Input: part model. Units: mm. Frame: model coordinates. A direction names the side the tool comes from. Give positions to 0.01 mm unless a question says otherwise; leave off trailing zeros. Write each loop counter-clockwise with the first axis right and the second up, starting at its lowest first coordinate (ties: lowest second). Pieces come first, ordered by that corner, then holes. Notation, with made-up numbers: (85, 30.5) - (106, 30.5) arc R15 ccw to (106, 50.5) - close; hole circle Ø8 at (70.5, -25). An arc over 180 degrees is marked (long way). Answer as CSV lines item,"result".
```python
from build123d import *

# Parameters (mm, degrees)
SKETCH1_R           = 6
BOSS_EXTRUDE1_DEPTH = 10
SKETCH2_W           = 6.574952472
SKETCH2_H           = 6.574952471
BOSS_EXTRUDE2_DEPTH = 60
CUT_EXTRUDE1_DEPTH  = 72.85269654


with BuildPart() as part:
    # Sketch1 → Boss-Extrude1 (new body)
    with BuildSketch(Plane(origin=(0, 0, 0), x_dir=(1, 0, 0), z_dir=(0, 1, 0))):
        with Locations(Location((0, 0, 0), (0, 0, 270))):
            Circle(SKETCH1_R)
        with BuildLine():
            Line((-3.287476236, 2.45), (3.287476236, 2.45))
            ThreePointArc((3.287476236, 2.45), (0, -4.1), (-3.287476236, 2.45))
        make_face(mode=Mode.SUBTRACT)
    boss_extrude1 = extrude(amount=BOSS_EXTRUDE1_DEPTH)

    # Sketch2 → Boss-Extrude2 (add)
    with BuildSketch(Plane.XY.offset(-2.45)):
        with Locations((0, 3.287476236)):
            Rectangle(SKETCH2_W, SKETCH2_H)
    extrude(amount=-BOSS_EXTRUDE2_DEPTH)

    # Mirror1: Boss-Extrude1 across plane
    add(boss_extrude1.mirror(Plane(origin=(0, 0, -32.45), x_dir=(1, 0, 0), z_dir=(0, 0, -1))))

    # Sketch3 → Cut-Extrude1 (cut, through all)
    with BuildSketch(Plane(origin=(0, 10, 0), x_dir=(1, 0, 0), z_dir=(0, 1, 0))):
        with BuildLine():
            Line((-3.297499052, 62.43), (3.297499052, 62.43))
            ThreePointArc((3.297499052, 62.43), (0, 69.02), (-3.297499052, 62.43))
        make_face()
    extrude(amount=-CUT_EXTRUDE1_DEPTH, mode=Mode.SUBTRACT)


solid = part.part
```
Item 1: Contact query for flat-ended pins moving along their axis: pin 1 (1 mm diameter, centred on y = 6, z = -17, fed in from -X); pin 2 (5 mm diameter, centred on x = 1, z = -23.5, fed in from +Y); pin 3 (5.5 mm diameter, centred on y = 2, z = -43.5, fed in from +X). Output: stop coordinate, or through.
The answers:
pin 1,"x = -3.29"
pin 2,"y = 6.57"
pin 3,"x = 3.29"
Item 2: Reachability of faces 3 (the face through (3.287, 3, -32)), 4 (the face through (0, 5, -62.43)), 5 (the face through (-3.287, 3, -32)) from +Z, -Z, +X, -X, +Y, -Y: full face, straight path, thin tool, end or side. Return the list, or none.
The answers:
face 3,"+X, +Y, -Y"
face 4,"+Y, -Y"
face 5,"-X, +Y, -Y"
Item 3: Ray query, line 1 (Z direction, x = 0.25, y = 7.75); line 2 (X direction, y = 5.5, z = 0); line 3 (Z direction, x = 1.5, y = 2.5). Return the intervals inside material, ascending. Write a range as from..to.
The answers:
line 1,"-70.89..-69.01, -62.43..-58.91, -5.99..-2.45, 4.09..5.99"
line 2,"-6..-4.1, 4.1..6"
line 3,"-70.71..-68.74, -62.43..-2.45, 3.82..5.81"
Item 4: Cut plane A-A on z = -64.9. Return the cut outline in (x, y).
The answers:
outline,"(-6, 0) - (-4.12, 0) - (-4.12, 10) - (-6, 10) - close; (4.12, 0) - (6, 0) - (6, 10) - (4.12, 10) - close"
Item 5: Mould query, pull axis Z, two halves, no side actions, for faces 1 (the face through (0.128, 5.07, -69.018)), 2 (the face through (0, 10, -62)). Classes: +Z half, -Z half, draft (parallel to the pull), parting line (faces both ways), or undercut.
The answers:
face 1,"undercut"
face 2,"draft"
Item 6: Cut plane C-C on x = 0. Return the cut outline in (y, z).
The answers:
outline,"(0, -70.9) - (10, -70.9) - (10, -69.02) - (0, -69.02) - close; (0, -62.43) - (10, -62.43) - (10, -58.9) - (6.57, -58.9) - (6.57, -6) - (10, -6) - (10, -2.45) - (0, -2.45) - close; (0, 4.1) - (10, 4.1) - (10, 6) - (0, 6) - close"
Item 7: Cut plane B-B on y = 1.25. Return the cut outline in (x, z), plus the area to 3 significant figures.
The answers:
outline,"(-3.29, -59.88) arc R6 ccw (long way) to (3.29, -59.88) - (3.29, -5.02) arc R6 ccw (long way) to (-3.29, -5.02) - close; hole (-3.3, -62.43) arc R4.12 ccw (long way) to (3.3, -62.43) - close; hole (-3.29, -2.45) - (3.29, -2.45) arc R4.1 ccw (long way) to start"
area,"487 mm²"
Item 8: Cut plane D-D on z = 0. Return the cut outline in (x, y).
The answers:
outline,"(-6, 0) - (-4.1, 0) - (-4.1, 10) - (-6, 10) - close; (4.1, 0) - (6, 0) - (6, 10) - (4.1, 10) - close"
